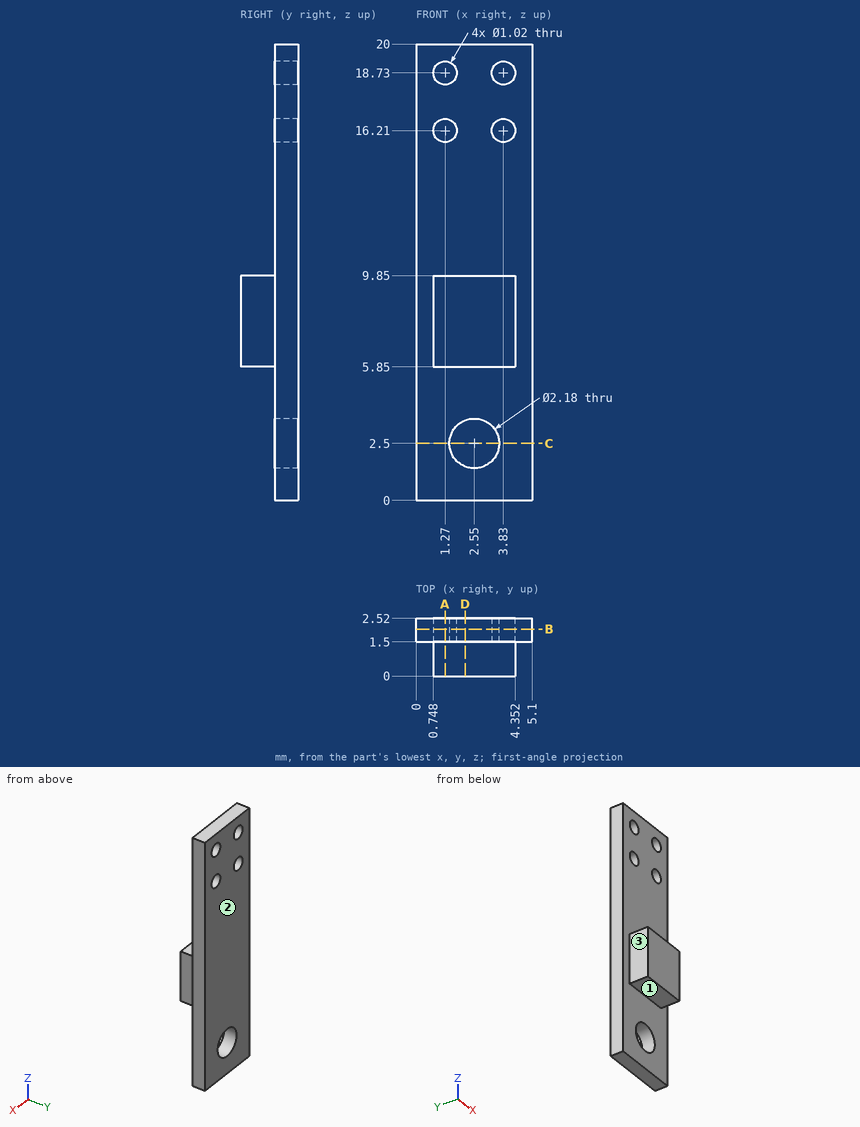
Can you work these out from the drawing? Everything is in mm from the part's minimum corner. A direction names the side the tool comes from. Give positions to 0.01 mm unless a question says otherwise; leave off trailing zeros. Order: outer loops, then holes, each group sorted by start corner. A loop starts at its lowest first (then second) coordinate and runs counter-clockwise, first axis right, second up. Notation, with made-up numbers: M 66.25,66 L 119.25,66 A13 cw 119.25,83 Z; hole C 5.25,-16.5 d3. An arc over 180 degrees is marked long. One line per question, with ' | ' between items.
1. If I drill on line 1 (Z direction, x = 1.27, y = 1.8); line 2 (X direction, y = 2.35, z = 16.21); line 3 (X direction, y = 1.9, z = 2.5), over which ranges is the centre line in solid material (lowest first)?
Results:
line 1: 0 to 15.7, 16.72 to 18.22, 19.24 to 20 | line 2: 0 to 0.76, 1.78 to 3.32, 4.34 to 5.1 | line 3: 0 to 1.46, 3.64 to 5.1
2. I want a section at B-B (y = 2.05). List the corners of the cut face in (x, z) for me.
Results:
outline: M 0,0 L 5.1,0 L 5.1,20 L 0,20 Z; hole C 1.27,16.21 d1.02; hole C 1.27,18.73 d1.02; hole C 2.55,2.5 d2.18; hole C 3.83,16.21 d1.02; hole C 3.83,18.73 d1.02
3. I want a section at C-C (z = 2.5). List the corners of the cut face in (x, y) for me.
Results:
outline: M 0,1.5 L 1.46,1.5 L 1.46,2.52 L 0,2.52 Z; M 3.64,1.5 L 5.1,1.5 L 5.1,2.52 L 3.64,2.52 Z
4. For the marked faces 1, 2 and 3, which set-ups out of +Z, -Z, +X, -X, +Y, -Y let a thin tool reach every point of the face, with its end or its side?
Results:
face 1: -Z, +X, -X, -Y | face 2: +Z, -Z, +X, -X, +Y | face 3: +Z, -Z, -X, -Y
5. I want a section at A-A (x = 1.27). List the corners of the cut face in (y, z) for me.
Results:
outline: M 0,5.85 L 1.5,5.85 L 1.5,0 L 2.52,0 L 2.52,15.7 L 1.5,15.7 L 1.5,9.85 L 0,9.85 Z; M 1.5,16.72 L 2.52,16.72 L 2.52,18.22 L 1.5,18.22 Z; M 1.5,19.24 L 2.52,19.24 L 2.52,20 L 1.5,20 Z
6. I'm going to push flat-ended pins straight in: pin 1 (2.5 mm diameter, centred on x = 3, z = 12.5, fed in from -Y); pin 2 (1.2 mm diameter, centred on y = 0.5, z = 8.5, fed in from -X); pin 3 (0.8 mm diameter, centred on x = 3, y = 0.5, fed in from +Z). Where does each tip first touch, or does it pass through?
Results:
pin 1: y = 1.5 | pin 2: x = 0.75 | pin 3: z = 9.85
7. I want a section at D-D (x = 2.15). List the corners of the cut face in (y, z) for me.
Results:
outline: M 0,5.85 L 1.5,5.85 L 1.5,3.51 L 2.52,3.51 L 2.52,20 L 1.5,20 L 1.5,9.85 L 0,9.85 Z; M 1.5,0 L 2.52,0 L 2.52,1.49 L 1.5,1.49 Z
